Read the model definition and answer for the solid it produces. Units are mm, in the model's axes. Face numbers are marked on the shaded views. A direction names the side the tool comes from. Coordinates: 2 decimals unless noted, no trailing zeros. Write each loop counter-clockwise with the first axis right and the second up, starting at its lowest first coordinate (ties: lowest second). Pieces come first, ordered by that corner, then holes. Notation, with made-up numbers: (40.5, 67) -> (95.5, 67) arc R32 cw to (95.5, 106) -> close; hole circle Ø7 at (-38, 8). An arc over 180 degrees is marked (long way). Answer in a Markdown table with one row per item. Add a question column.
Item 1: Which of the six approach directions +Z, -Z, +X, -X, +Y, -Y give full straight-line access (tool end or side, diameter ignored) to the marked faces 1, 2 and 3?
Item 2: Section A-A on z = -23 is taken. Write down the section's boundary in (x, y).
Item 3: Section D-D on y = 23.5 is taken. Write down the section's boundary in (x, z).
Item 4: Section B-B on x = 4.75 is taken. Write down the section's boundary in (y, z), then the cut area to 3 significant figures.
Item 5: Section C-C on x = 1 is taken. Write down the section's boundary in (y, z), then the cut area to 3 significant figures.
Item 6: Straight lines are drawn through the part: line 1 (Z direction, x = 8.75, y = 3.5); line 2 (Y direction, x = 2.25, z = -37.5); line 3 (Z direction, x = 13.75, y = 31.5). For each, find the intervals that lie inside material, in ascending order. Write a range as from..to.
Item 7: For a pull along X with two mould halves and no side action, classify the marked faces 4, 5 and 6 as +X half, -X half, draft (parallel to the pull), parting line (faces both ways), or undercut.
Item 8: Given pin 1 Ø4 at (x, y) = (9, 23) entering from -Z; pin 2 Ø5 at (x, y) = (12.5, 27) entering from +Z, each flat-ended and moving along its own axis, determine where each tip first touches the part or whether it passes through.
```python
from build123d import *

# Parameters (mm, degrees)
SKETCH1_R           = 2.328333333
BOSS_EXTRUDE1_DEPTH = 14.2875
SKETCH2_R           = 3.175
CUT_EXTRUDE1_DEPTH  = 14.2875


with BuildPart() as part:
    # Sketch1 → Boss-Extrude1 (new body)
    with BuildSketch(Plane(origin=(0, 0, 0), x_dir=(0, 0, -1), z_dir=(1, 0, 0))):
        Polygon((0, 0), (42.8625, 0), (42.8625, 6.35), (30.1625, 6.35), (30.1625, 33.3375), (12.7, 33.3375), (12.7, 6.35), (0, 6.35), align=None)
        with Locations((21.43125, 21.9075)):
            Circle(SKETCH1_R, mode=Mode.SUBTRACT)
    extrude(amount=BOSS_EXTRUDE1_DEPTH)

    # Sketch2 → Cut-Extrude1 (cut)
    with BuildSketch(Plane(origin=(0, 6.35, 0), x_dir=(1, 0, 0), z_dir=(0, 1, 0))):
        with Locations(Location((7.14375, 5.55625, 0), (0, 0, 270))):
            Circle(SKETCH2_R)
        with Locations(Location((7.14375, 37.30625, 0), (0, 0, 270))):
            Circle(SKETCH2_R)
    extrude(amount=-CUT_EXTRUDE1_DEPTH, mode=Mode.SUBTRACT)


solid = part.part
```
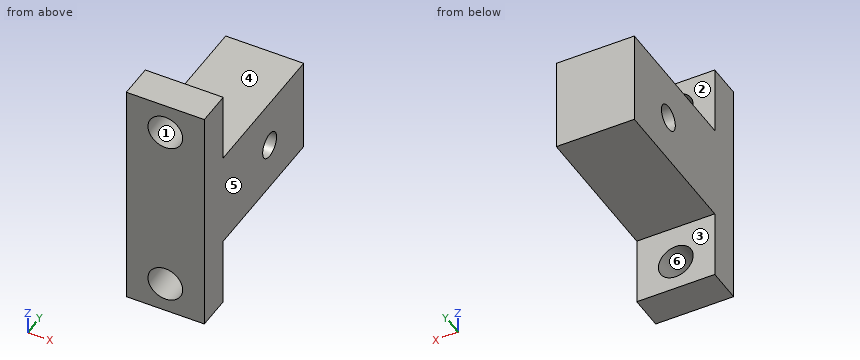
Results below:
| question | item | result |
|---|---|---|
| 1 | face 1 | +Y, -Y |
| 1 | face 2 | +Z, +X, -X, +Y |
| 1 | face 3 | -Z, +X, -X, +Y |
| 2 | outline | (0, 0) -> (14.29, 0) -> (14.29, 20.19) -> (0, 20.19) -> close; (0, 23.63) -> (14.29, 23.63) -> (14.29, 33.34) -> (0, 33.34) -> close |
| 3 | outline | (0, -30.16) -> (14.29, -30.16) -> (14.29, -23.13) -> (0, -23.13) -> close; (0, -19.73) -> (14.29, -19.73) -> (14.29, -12.7) -> (0, -12.7) -> close |
| 4 | outline | (0, -42.86) -> (6.35, -42.86) -> (6.35, -39.39) -> (0, -39.39) -> close; (0, -35.22) -> (6.35, -35.22) -> (6.35, -30.16) -> (33.34, -30.16) -> (33.34, -12.7) -> (6.35, -12.7) -> (6.35, -7.64) -> (0, -7.64) -> close; (0, -3.47) -> (6.35, -3.47) -> (6.35, 0) -> (0, 0) -> close; hole circle Ø4.66 at (21.91, -21.43) |
| 4 | area | 673 mm2 |
| 5 | outline | (0, -42.86) -> (6.35, -42.86) -> (6.35, -30.16) -> (33.34, -30.16) -> (33.34, -12.7) -> (6.35, -12.7) -> (6.35, 0) -> (0, 0) -> close; hole circle Ø4.66 at (21.91, -21.43) |
| 5 | area | 726 mm2 |
| 6 | line 1 | z = -42.86..-40.04, -34.57..-8.29, -2.82..0 |
| 6 | line 2 | y = 0..6.35 |
| 6 | line 3 | z = -30.16..-12.7 |
| 7 | face 4 | draft |
| 7 | face 5 | +X half |
| 7 | face 6 | undercut |
| 8 | pin 1 | stops at z = -30.16 |
| 8 | pin 2 | stops at z = -12.7 |
